Read the model definition and answer for the solid it produces. Units are mm, in the model's axes. A direction names the side the tool comes from. Coordinates: 2 decimals unless noted, no trailing zeros. Loops run counter-clockwise (first coordinate to the right, second up) from the corner with the lowest first, then second, coordinate; pieces in that order, holes last.
from build123d import *

# Parameters (mm, degrees)
BOSS_EXTRUDE1_DEPTH = 10
FILLET1_R           = 10
FILLET2_R           = 3
SKETCH5_R           = 10
BOSS_EXTRUDE2_DEPTH = 10
SKETCH4_R           = 2.75
CUT_EXTRUDE1_DEPTH  = 10
BOSS_EXTRUDE3_DEPTH = 10


with BuildPart() as part:
    # Sketch1 → Boss-Extrude1 (new body)
    with BuildSketch(Plane(origin=(0, 0, 0), x_dir=(1, 0, 0), z_dir=(0, 1, 0))):
        Polygon((-81.738081939, 0), (0, 171.628518507), (81.738081939, 0), align=None)
        Polygon((0, 148.371481493), (-67.328168061, 7), (67.328168061, 7), align=None, mode=Mode.SUBTRACT)
    extrude(amount=BOSS_EXTRUDE1_DEPTH)

    # Fillet1
    fillet1_edges = [part.edges().sort_by_distance(p)[0] for p in [
        (0, 5, -171.628518507),
    ]]
    fillet(fillet1_edges, radius=FILLET1_R)

    # Fillet2
    fillet2_edges = [part.edges().sort_by_distance(p)[0] for p in [
        (0, 5, -148.371481493),
        (-67.328168061, 5, -7),
        (67.328168061, 5, -7),
    ]]
    fillet(fillet2_edges, radius=FILLET2_R)

    # Sketch5 → Boss-Extrude2 (add, through all)
    with BuildSketch(Plane(origin=(0, 10, 0), x_dir=(1, 0, 0), z_dir=(0, 1, 0))):
        with Locations((0, 148.371481493)):
            Circle(SKETCH5_R)
    extrude(amount=-BOSS_EXTRUDE2_DEPTH)

    # Sketch4 → Cut-Extrude1 (cut)
    with BuildSketch(Plane(origin=(0, 10, 0), x_dir=(1, 0, 0), z_dir=(0, 1, 0))):
        with Locations((0, 148.371481493)):
            Circle(SKETCH4_R)
    extrude(amount=-CUT_EXTRUDE1_DEPTH, mode=Mode.SUBTRACT)

    # Sketch6 → Boss-Extrude3 (add, through all)
    with BuildSketch(Plane(origin=(0, 10, 0), x_dir=(1, 0, 0), z_dir=(0, 1, 0))):
        with BuildLine():
            Line((-26.19375, 93.371481493), (0, 124.587977159))
            Line((0, 124.587977159), (26.19375, 93.371481493))
            Line((26.19375, 93.371481493), (4.299773868, 139.34308492))
            ThreePointArc((4.299773868, 139.34308492), (0, 138.371481493), (-4.299773868, 139.34308492))
            Line((-4.299773868, 139.34308492), (-26.19375, 93.371481493))
        make_face()
    extrude(amount=-BOSS_EXTRUDE3_DEPTH)


solid = part.part
Q1. Which of the six approach directions +Z, -Z, +X, -X, +Y, -Y give full straight-line access (tool end or side, diameter ignored) to faces 4 (the face through (12.91, 5.07, -109.2)), 5 (the face through (-45.89, 4.93, -75.27))?
Findings below:
face 4: +Y, -Y
face 5: -Z, -X, +Y, -Y
Q2. Determine the mould class of faces 1 (the face through (-0.16, 5.07, -158.37)), 2 (the face through (-31, 0, -85)), 3 (the face through (46.01, 4.93, -51.76)) for opening direction Z: +Z half, -Z half, draft (parallel to the pull), parting line (faces both ways), or undercut.
Findings below:
face 1: -Z half
face 2: draft
face 3: undercut
Q3. A cutting plane is placed at C-C (y = 4.5). Give the vertices of the cut face in (x, z).
Findings below:
outline: (-81.74, 0) - (-9.03, -152.67) arc R10 ccw to (9.03, -152.67) - (81.74, 0) - close; hole (-65.29, -11.29) - (-26.19, -93.37) - (0, -124.59) - (26.19, -93.37) - (65.29, -11.29) arc R3 ccw to (62.58, -7) - (-62.58, -7) arc R3 ccw to start; hole circle Ø5.5 at (0, -148.37)
Q4. A cutting plane is placed at B-B (x = -19.5). Give the vertices of the cut face in (y, z), then the cut area to 3 significant figures.
Findings below:
outline: (0, -130.68) - (10, -130.68) - (10, -101.35) - (0, -101.35) - close; (0, -7) - (10, -7) - (10, 0) - (0, 0) - close
area: 363 mm2
Q5. A flat-ended cylindrical pin translates along its axis: pin 1 Ø5 at (y, z) = (8.5, -72.5) entering from -X. Find the tip coordinate at first contact, or state that the pin passes through.
Findings below:
pin 1: stops at x = -48.4
Q6. Straight lines are drawn through the part: probe 1 along Z at (x, y) = (0, 4.25); probe 2 along X at (y, z) = (1, -40); probe 3 along X at (y, z) = (1.75, -51). For each, find the intervals that lie inside material, in ascending order.
Findings below:
probe 1: z = -158.37 to -151.12, -145.62 to -124.59, -7 to 0
probe 2: x = -62.69 to -51.61, 51.61 to 62.69
probe 3: x = -57.45 to -46.37, 46.37 to 57.45
Q7. A cutting plane is placed at A-A (z = -122). Give the vertices of the cut face in (x, y).
Findings below:
outline: (-23.64, 0) - (-2.17, 0) - (-2.17, 10) - (-23.64, 10) - close; (2.17, 0) - (23.64, 0) - (23.64, 10) - (2.17, 10) - close
